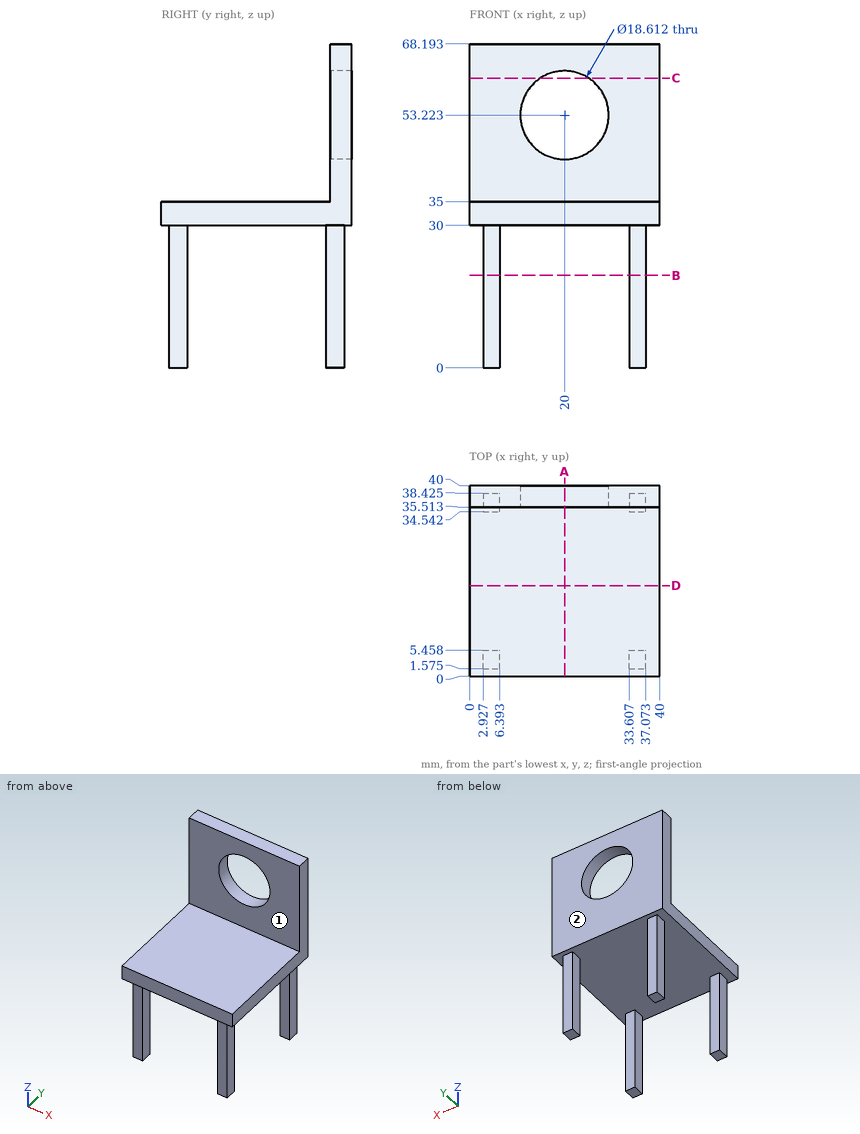
For this review, use the dimensioned drawing (mm, ordinates from the lowest corner) and the shaded views. A direction names the side the tool comes from. Coordinates: 2 decimals unless noted, no trailing zeros. Write each loop counter-clockwise with the first axis right and the second up, starting at its lowest first coordinate (ties: lowest second). Pieces come first, ordered by that corner, then holes. Notation, with made-up numbers: (68, 85) - (106, 85) arc R15 cw to (106, 103) - close; hole circle Ø7 at (0, 63.5). An arc over 180 degrees is marked (long way). Answer as a JSON object with one key per item and string values. Group by question number.
1. Clearance check with flat-ended pins moving along their axes: pin 1 Ø1 at (x, z) = (5, 21) entering from +Y (1 decimal); pin 2 Ø4 at (x, y) = (4.5, 16.5) entering from +Z; pin 3 Ø1.9 at (y, z) = (36, 19.5) entering from +X. State where each tip first meets the part, or that it passes through.
2. Add section C-C (z = 61). Give the boundary of the cut face in (x, y), plus the area to 3 significant figures.
3. Add section A-A (x = 20). Give the boundary of the cut face in (y, z).
4. Machinability: for the marked faces 1 and 2, which of the approach directions +Z, -Z, +X, -X, +Y, -Y give a long, thin tool a straight path to every point of the face, cutting with its end or side? Answer none if there is none.
5. Add section D-D (y = 19). Give the boundary of the cut face in (x, z), plus the area to 3 significant figures.
6. To check wall thickness, follow probe 1 along X at (y, z) = (3, 15.5); probe 2 along Z at (x, y) = (20, 37.85); probe 3 along Z at (x, y) = (10, 28). State the ranges of each line that lie inside material, in increasing order.
7. Add section B-B (z = 19.5). Give the boundary of the cut face in (x, y) (1 decimal).
Findings:
{
 "1": {"pin 1": "y = 38.4", "pin 2": "z = 35", "pin 3": "x = 37.07"},
 "2": {"outline": "(0, 35.51) - (14.89, 35.51) - (14.89, 40) - (0, 40) - close; (25.11, 35.51) - (40, 35.51) - (40, 40) - (25.11, 40) - close", "area": "134 mm²"},
 "3": {"outline": "(0, 30) - (40, 30) - (40, 43.92) - (35.51, 43.92) - (35.51, 35) - (0, 35) - close; (35.51, 62.53) - (40, 62.53) - (40, 68.19) - (35.51, 68.19) - close"},
 "4": {"face 1": "+Z, +X, -X, -Y", "face 2": "+Z, -Z, +X, -X, +Y"},
 "5": {"outline": "(0, 30) - (40, 30) - (40, 35) - (0, 35) - close", "area": "200 mm²"},
 "6": {"probe 1": "2.93 to 6.39, 33.61 to 37.07", "probe 2": "30 to 43.92, 62.53 to 68.19", "probe 3": "30 to 35"},
 "7": {"outline": "(2.9, 1.6) - (6.4, 1.6) - (6.4, 5.5) - (2.9, 5.5) - close; (2.9, 34.5) - (6.4, 34.5) - (6.4, 38.4) - (2.9, 38.4) - close; (33.6, 1.6) - (37.1, 1.6) - (37.1, 5.5) - (33.6, 5.5) - close; (33.6, 34.5) - (37.1, 34.5) - (37.1, 38.4) - (33.6, 38.4) - close"}
}
